Verification items for the finished model (mm, model axes). A direction names the side the tool comes from. Round coordinates to 2 decimals unless told otherwise and drop trailing zeros. Write each loop counter-clockwise with the first axis right and the second up, starting at its lowest first coordinate (ties: lowest second). Pieces come first, ordered by that corner, then holes. Notation, with made-up numbers: (34, 56) - (50, 56) arc R24 ccw to (50, 79) - close; hole circle Ø2 at (-32.75, 88). An arc over 180 degrees is marked (long way). Answer as a JSON object with one key per item and string values.
```python
from build123d import *

# Parameters (mm, degrees)
BOSS_EXTRUDE1_DEPTH                             = 12
SKETCH2_R                                       = 22.5
CUT_EXTRUDE1_DEPTH                              = 5
SKETCH3_R                                       = 2.5
CUT_EXTRUDE2_DEPTH                              = 94.45587194
CIRPATTERN1_COUNT                               = 5
SKETCH4_R                                       = 1.25
CUT_EXTRUDE3_DEPTH                              = 94.96275858
CIRPATTERN2_COUNT                               = 4
SKETCH11_R                                      = 3.5
CUT_EXTRUDE8_DEPTH                              = 14.5
SKETCH13_R                                      = 3.25
CUT_EXTRUDE9_DEPTH                              = 8
LPATTERN2_COUNT                                 = 2
LPATTERN2_PITCH                                 = 28.2
SKETCH14_R                                      = 2.5
CUT_EXTRUDE10_DEPTH                             = 8
LPATTERN3_COUNT                                 = 3
LPATTERN3_PITCH                                 = 23
CSK_FOR_M5_FLAT_HEAD_MACHINE_SCREW1_D           = 5
CSK_FOR_M5_FLAT_HEAD_MACHINE_SCREW1_CSINK_D     = 9
CSK_FOR_M5_FLAT_HEAD_MACHINE_SCREW1_CSINK_ANGLE = 90


with BuildPart() as part:
    # Sketch1 → Boss-Extrude1 (new body)
    with BuildSketch(Plane.XY):
        with BuildLine():
            Line((45, 30), (51, 30))
            ThreePointArc((51, 30), (3, 78), (-45, 30))
            Line((-45, 30), (-45, -30))
            Line((-45, -30), (45, -30))
            Line((45, -30), (45, 30))
        make_face()
    extrude(amount=BOSS_EXTRUDE1_DEPTH)

    # Sketch2 → Cut-Extrude1 (cut)
    with BuildSketch(Plane.XY.offset(12)):
        with Locations((3, 30)):
            Circle(SKETCH2_R)
    extrude(amount=-CUT_EXTRUDE1_DEPTH, mode=Mode.SUBTRACT)

    # Sketch3 → Cut-Extrude2 (cut, through all)
    with BuildSketch(Plane.XY.offset(7)):
        with Locations((3.751645972, 47.483850501)):
            Circle(SKETCH3_R)
    cut_extrude2 = extrude(amount=-CUT_EXTRUDE2_DEPTH, mode=Mode.SUBTRACT)

    # CirPattern1: Cut-Extrude2 ×5 about axis
    cirpattern1_axis = Axis((3, 30, 0), (0, 0, 1))
    for i in range(1, CIRPATTERN1_COUNT):
        add(cut_extrude2.rotate(cirpattern1_axis, i * 360 / CIRPATTERN1_COUNT), mode=Mode.SUBTRACT)

    # Sketch4 → Cut-Extrude3 (cut, through all)
    with BuildSketch(Plane.XY.offset(12)):
        with Locations((3, 56.81356815)):
            Circle(SKETCH4_R)
    cut_extrude3 = extrude(amount=-CUT_EXTRUDE3_DEPTH, mode=Mode.SUBTRACT)

    # CirPattern2: Cut-Extrude3 ×4 about axis
    cirpattern2_axis = Axis((3, 30, 0), (0, 0, 1))
    for i in range(1, CIRPATTERN2_COUNT):
        add(cut_extrude3.rotate(cirpattern2_axis, i * 360 / CIRPATTERN2_COUNT), mode=Mode.SUBTRACT)

    # Sketch11 → Cut-Extrude8 (cut)
    with BuildSketch(Plane.XY.offset(12)):
        with Locations((20, -20)):
            Circle(SKETCH11_R)
    extrude(amount=-CUT_EXTRUDE8_DEPTH, mode=Mode.SUBTRACT)

    # Sketch13 → Cut-Extrude9 (cut)
    with BuildSketch(Plane.XZ.offset(30)):
        with Locations(Location((-36.7, 5.2, 0), (0, 0, 270))):
            Circle(SKETCH13_R)
    cut_extrude9 = extrude(amount=-CUT_EXTRUDE9_DEPTH, mode=Mode.SUBTRACT)

    # LPattern2: Cut-Extrude9 ×2
    with Locations(*[(i * LPATTERN2_PITCH, 0, 0) for i in range(1, LPATTERN2_COUNT)]):
        add(cut_extrude9, mode=Mode.SUBTRACT)

    # Sketch14 → Cut-Extrude10 (cut)
    with BuildSketch(Plane(origin=(45, 0, 0), x_dir=(0, 0, -1), z_dir=(1, 0, 0))):
        with Locations((-6, -23)):
            Circle(SKETCH14_R)
    cut_extrude10 = extrude(amount=-CUT_EXTRUDE10_DEPTH, mode=Mode.SUBTRACT)

    # LPattern3: Cut-Extrude10 ×3
    with Locations(*[(0, i * LPATTERN3_PITCH, 0) for i in range(1, LPATTERN3_COUNT)]):
        add(cut_extrude10, mode=Mode.SUBTRACT)

    # CSK for M5 Flat Head Machine Screw1 (through all)
    with Locations(Plane.XY.offset(12)):
        with Locations((-39, 24.3), (-39, 0.3), (-24, 16.3)):
            CounterSinkHole(CSK_FOR_M5_FLAT_HEAD_MACHINE_SCREW1_D / 2, CSK_FOR_M5_FLAT_HEAD_MACHINE_SCREW1_CSINK_D / 2, counter_sink_angle=CSK_FOR_M5_FLAT_HEAD_MACHINE_SCREW1_CSINK_ANGLE)


solid = part.part
```
Q1. Release check for a two-part mould opening along X. For faces 1 (the cylindrical face through (41.056, 0.751, 3.615)), 2 (the flat face through (37, 0, 6)), 3 (the cylindrical face through (-41.31, 23.34, 4.93)) record: released by +X, released by -X, zero draft, split by the parting line, or undercut.
Geometry check:
{"face 1": "zero draft", "face 2": "released by +X", "face 3": "undercut"}
Q2. Material ranges on line 1 along Y through (x, z) = (3, 10.5); line 2 along Y through (x, z) = (3, 4); line 3 along X through (y, z) = (16.3, 7.75), recorded low to high. Write a range as [from, to].
Geometry check:
{"line 1": "y = [-30, 1.94], [4.44, 7.5], [52.5, 55.56], [58.06, 78]", "line 2": "y = [-30, 1.94], [4.44, 45.1], [49.87, 55.56], [58.06, 78]", "line 3": "x = [-45, -26.5], [-21.5, -14.85], [20.85, 45]"}
Q3. Section check C-C, the plane y = 63. Record the cut outline in (x, z).
Geometry check:
{"outline": "(-31.86, 0) - (37.86, 0) - (37.86, 12) - (-31.86, 12) - close"}
Q4. Section check A-A, the plane y = 16.3. Record the cut outline in (x, z).
Geometry check:
{"outline": "(-45, 0) - (-26.5, 0) - (-26.5, 10) - (-28.5, 12) - (-45, 12) - close; (-21.5, 0) - (-10.38, 0) - (-10.38, 7) - (-14.85, 7) - (-14.85, 12) - (-19.5, 12) - (-21.5, 10) - close; (-5.38, 0) - (10.33, 0) - (10.33, 7) - (-5.38, 7) - close; (15.01, 0) - (45, 0) - (45, 12) - (20.85, 12) - (20.85, 7) - (15.01, 7) - close"}
Q5. Section check B-B, the plane x = 35.5. Record the cut outline in (y, z).
Geometry check:
{"outline": "(-30, 0) - (65.32, 0) - (65.32, 12) - (-30, 12) - close"}
Q6. Set-up check for faces 4 (the cylindrical face through (-41.31, -0.66, 4.93)), 5 (the cylindrical face through (41.06, -20.89, 4.66)), 6 (the cylindrical face through (-9.745, -26.056, 2.198)), 7 (the flat face through (2, 25, 0)), 8 (the flat face through (48, 30, 6)): record each of +Z, -Z, +X, -X, +Y, -Y from which the full face is reachable in a straight line by a thin tool's end or side.
Geometry check:
{"face 4": "+Z, -Z", "face 5": "+X", "face 6": "-Y", "face 7": "-Z, +X, -X, +Y, -Y", "face 8": "+Z, -Z, +X, -Y"}
Q7. Gauge pin test, flat ends, axial feed: P1, Ø5, axis at x = -7.5, z = 5, coming from the -Y side; P2, Ø6, axis at x = -13.4, y = 36.12, coming from the +Z side; P3, Ø2.5, axis at y = -22, z = 7, coming from the +X side; P4, Ø4, axis at x = -8.5, z = 6.5, coming from the +Y side. Record the tip position at first contact, or that the pin passes through.
Geometry check:
{"P1": "stops at y = -30", "P2": "stops at z = 7", "P3": "stops at x = 45", "P4": "stops at y = 77.05"}
